Can you work these out from the model? Positions are in its coordinate system, mm. Face numbers are marked on the shaded views. A direction names the side the tool comes from. Round coordinates to 2 decimals unless told otherwise and drop trailing zeros. Write each loop counter-clockwise with the first axis right and the second up, starting at its lowest first coordinate (ties: lowest second). Pieces come first, ordered by that corner, then holes.
Q1. If we section it at B-B (x = -33): Please give me the cut outline in (y, z).
Q2. For the marked faces 3 and 4, which set-ups out of +Z, -Z, +X, -X, +Y, -Y let a thin tool reach every point of the face, with its end or its side?
Q3. We'd pull the mould along X, two halves only. Please class the marked faces 1 and 2: +X half, -X half, draft (parallel to the pull), parting line (faces both ways), or undercut.
Q4. If we section it at C-C (x = -18.5): Please give me the cut outline in (y, z).
Q5. Please list where these lines run through material, in increasing order: line 1 along Y through (x, z) = (-33, 3); line 2 along Y through (x, z) = (33, 2.75); line 3 along Z through (x, y) = (26, 29).
Q6. If we section it at A-A (y = -19.5): Please give me the cut outline in (x, z), plus the area to 3 significant figures.
Q7. I'm going to push flat-ended pins straight in: pin 1 Ø3.5 at (y, z) = (26, 3.5) entering from -X; pin 2 Ø10 at (x, y) = (34.5, 16.5) entering from +Z; pin 3 Ø1.8 at (x, y) = (33, 26.5) entering from +Z; pin 4 Ø5 at (y, z) = (12, -3) entering from -X. Where does each tip first touch, or does it pass through?
Q8. If we section it at D-D (y = 15.5): Please give me the cut outline in (x, z).
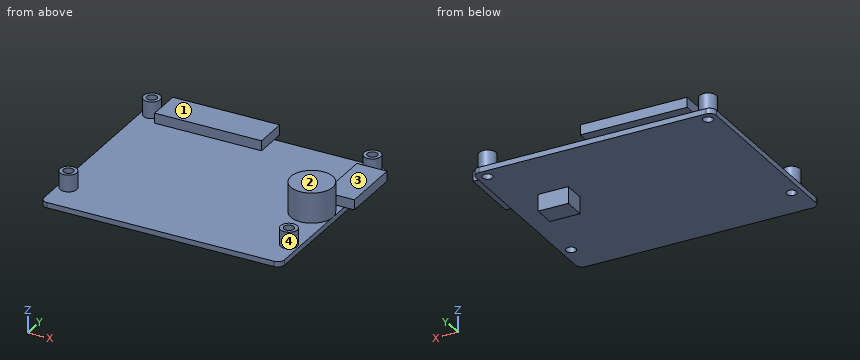
from build123d import *

# Parameters (mm, degrees)
SKETCH_1_R      = 1.5
EXTRUDE_1_DEPTH = 1.6
SKETCH_2_R      = 2.5
SKETCH_2_R_2    = 1.5
EXTRUDE_2_DEPTH = 5
SKETCH_3_R      = 6.3
EXTRUDE_3_DEPTH = 9
EXTRUDE_4_DEPTH = 3
SKETCH_5_W      = 9
SKETCH_5_H      = 6.5
EXTRUDE_5_DEPTH = 5


with BuildPart() as part:
    # 草图1 → 凸台-拉伸1 (new body)
    with BuildSketch(Plane.XY):
        with BuildLine():
            Line((-34, -29.5), (34, -29.5))
            ThreePointArc((34, -29.5), (35.414213562, -28.914213562), (36, -27.5))
            Line((36, -27.5), (36, 27.5))
            ThreePointArc((36, 27.5), (35.414213562, 28.914213562), (34, 29.5))
            Line((34, 29.5), (-34, 29.5))
            ThreePointArc((-34, 29.5), (-35.414213562, 28.914213562), (-36, 27.5))
            Line((-36, 27.5), (-36, -27.5))
            ThreePointArc((-36, -27.5), (-35.414213562, -28.914213562), (-34, -29.5))
        make_face()
        with Locations((-33, 26.5)):
            Circle(SKETCH_1_R, mode=Mode.SUBTRACT)
        with Locations((33, 26.5)):
            Circle(SKETCH_1_R, mode=Mode.SUBTRACT)
        with Locations((33, -19.5)):
            Circle(SKETCH_1_R, mode=Mode.SUBTRACT)
        with Locations((-33, -19.5)):
            Circle(SKETCH_1_R, mode=Mode.SUBTRACT)
    extrude(amount=EXTRUDE_1_DEPTH)

    # 草图2 → 凸台-拉伸2 (add)
    # profile 1 of 4: a face of its own
    with BuildSketch(Plane.XY.offset(1.6)):
        with Locations(Location((33, 26.5, 0), (0, 0, 180))):
            Circle(SKETCH_2_R)
        with Locations((33, 26.5)):
            Circle(SKETCH_2_R_2, mode=Mode.SUBTRACT)
    # profile 2 of 4: a face of its own
    with BuildSketch(Plane.XY.offset(1.6)):
        with Locations(Location((-33, 26.5, 0), (0, 0, 180))):
            Circle(SKETCH_2_R)
        with Locations((-33, 26.5)):
            Circle(SKETCH_2_R_2, mode=Mode.SUBTRACT)
    # profile 3 of 4: a face of its own
    with BuildSketch(Plane.XY.offset(1.6)):
        with Locations(Location((-33, -19.5, 0), (0, 0, 180))):
            Circle(SKETCH_2_R)
        with Locations((-33, -19.5)):
            Circle(SKETCH_2_R_2, mode=Mode.SUBTRACT)
    # profile 4 of 4: a face of its own
    with BuildSketch(Plane.XY.offset(1.6)):
        with Locations(Location((33, -19.5, 0), (0, 0, 180))):
            Circle(SKETCH_2_R)
        with Locations((33, -19.5)):
            Circle(SKETCH_2_R_2, mode=Mode.SUBTRACT)
    extrude(amount=EXTRUDE_2_DEPTH)

    # 草图3 → 凸台-拉伸3 (add)
    with BuildSketch(Plane.XY.offset(1.6)):
        with Locations((29.7, -0.8)):
            Circle(SKETCH_3_R)
    extrude(amount=EXTRUDE_3_DEPTH)

    # 草图4 → 凸台-拉伸4 (add)
    with BuildSketch(Plane.XY.offset(1.6)):
        Polygon((36, 5.5), (30, 5.5), (30, 23.5), (36, 23.5), (39, 23.5), (39, 5.5), align=None)
        Polygon((2, 29.5), (2, 22.5), (-30, 22.5), (-30, 29.5), (-30, 32.5), (2, 32.5), align=None)
    extrude(amount=EXTRUDE_4_DEPTH)

    # 草图5 → 凸台-拉伸5 (add)
    with BuildSketch(Plane(origin=(0, 0, 0), x_dir=(-1, 0, 0), z_dir=(0, 0, -1))):
        with Locations((-21.5, 8.25)):
            Rectangle(SKETCH_5_W, SKETCH_5_H)
    extrude(amount=EXTRUDE_5_DEPTH)


solid = part.part
A:
1. outline: (-29.5, 0) - (-21, 0) - (-21, 6.6) - (-22, 6.6) - (-22, 1.6) - (-29.5, 1.6) - close; (-18, 0) - (25, 0) - (25, 6.6) - (24, 6.6) - (24, 1.6) - (-17, 1.6) - (-17, 6.6) - (-18, 6.6) - close; (28, 0) - (29.5, 0) - (29.5, 1.6) - (29, 1.6) - (29, 6.6) - (28, 6.6) - close
2. face 3: +Z, +X, -X
2. face 4: +Z
3. face 1: undercut
3. face 2: draft
4. outline: (-29.5, 0) - (29.5, 0) - (29.5, 1.6) - (32.5, 1.6) - (32.5, 4.6) - (22.5, 4.6) - (22.5, 1.6) - (-29.5, 1.6) - close
5. line 1: y = -22 to -21, -18 to -17, 24 to 25, 28 to 29
5. line 2: y = -22 to -21, -18 to -17, -6.17 to 4.57, 5.5 to 23.5, 24 to 25, 28 to 29
5. line 3: z = 0 to 1.6
6. outline: (-36, 0) - (-34.5, 0) - (-34.5, 6.6) - (-35.5, 6.6) - (-35.5, 1.6) - (-36, 1.6) - close; (-31.5, 0) - (31.5, 0) - (31.5, 6.6) - (30.5, 6.6) - (30.5, 1.6) - (-30.5, 1.6) - (-30.5, 6.6) - (-31.5, 6.6) - close; (34.5, 0) - (36, 0) - (36, 1.6) - (35.5, 1.6) - (35.5, 6.6) - (34.5, 6.6) - close
6. area: 126 mm2
7. pin 1: stops at x = -35.5
7. pin 2: stops at z = 4.6
7. pin 3: passes through
7. pin 4: stops at x = 17
8. outline: (-36, 0) - (36, 0) - (36, 1.6) - (39, 1.6) - (39, 4.6) - (30, 4.6) - (30, 1.6) - (-36, 1.6) - close
